Geometry: see drawing. Coordinates: mm, zero at the bounding-box minimum. A direction names the side the tool comes from. Round coordinates to 2 decimals unless told otherwise and drop trailing zeros. Order: outer loops, then holes, each group sorted by start corner. A loop starts at its lowest first (then second) coordinate and runs counter-clockwise, first axis right, second up. Notation, with made-up numbers: (21, 38.5) -> (43, 38.5) arc R14 ccw to (43, 58.5) -> close; hole circle Ø10 at (-16, 77.25). An arc over 180 degrees is marked (long way). Answer as CSV lines item,"result". Start each with the question number.
(1) Section query B-B (z = 7.5). Output: boundary loops of the cut face in (x, y), plus the area to 3 significant figures.
(2) Set-up query: the marked faces 1 and 2. Return all of +Z, -Z, +X, -X, +Y, -Y with unobstructed straight access to the full face (end or side cutting, diameter ignored); none if empty.
(3) Contact query for flat-ended pins moving along their axis: P1, Ø4.5, axis at y = 12.5, z = 9, coming from the +X side; P2, Ø4, axis at x = 97, y = 11.5, coming from the +Z side. Output: stop coordinate, or through.
(4) Section query D-D (y = 18). Output: boundary loops of the cut face in (x, z).
(5) Line query: line 1 along X through (y, z) = (21.5, 8.5); line 2 along Y through (x, z) = (8, 6); line 3 along Y through (x, z) = (8.5, 6.5). Output: solid intervals per line, ascending. Write a range as from..to.
(6) Section query C-C (x = 10.5). Output: boundary loops of the cut face in (y, z).
(7) Section query A-A (y = 8). Output: boundary loops of the cut face in (x, z), plus the area to 4 significant figures.
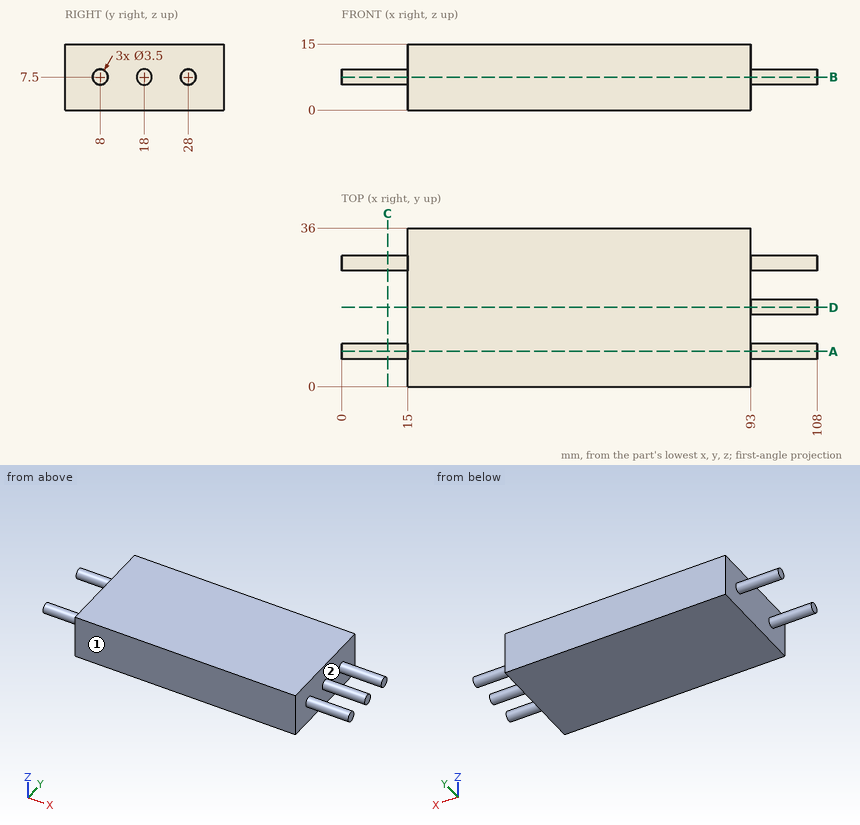
Answer block:
1,outline,"(0, 6.25) -> (15, 6.25) -> (15, 0) -> (93, 0) -> (93, 6.25) -> (108, 6.25) -> (108, 9.75) -> (93, 9.75) -> (93, 16.25) -> (108, 16.25) -> (108, 19.75) -> (93, 19.75) -> (93, 26.25) -> (108, 26.25) -> (108, 29.75) -> (93, 29.75) -> (93, 36) -> (15, 36) -> (15, 29.75) -> (0, 29.75) -> (0, 26.25) -> (15, 26.25) -> (15, 9.75) -> (0, 9.75) -> close"
1,area,"3,070 mm2"
2,face 1,"+Z, -Z, +X, -X, -Y"
2,face 2,"+X"
3,P1,"x = 93"
3,P2,"z = 8.4"
4,outline,"(15, 0) -> (93, 0) -> (93, 5.75) -> (108, 5.75) -> (108, 9.25) -> (93, 9.25) -> (93, 15) -> (15, 15) -> close"
5,line 1,"15..93"
5,line 2,"7.1..8.9, 27.1..28.9"
5,line 3,"6.56..9.44, 26.56..29.44"
6,outline,"circle Ø3.5 at (8, 7.5); circle Ø3.5 at (28, 7.5)"
7,outline,"(0, 5.75) -> (15, 5.75) -> (15, 0) -> (93, 0) -> (93, 5.75) -> (108, 5.75) -> (108, 9.25) -> (93, 9.25) -> (93, 15) -> (15, 15) -> (15, 9.25) -> (0, 9.25) -> close"
7,area,"1,275 mm2"
